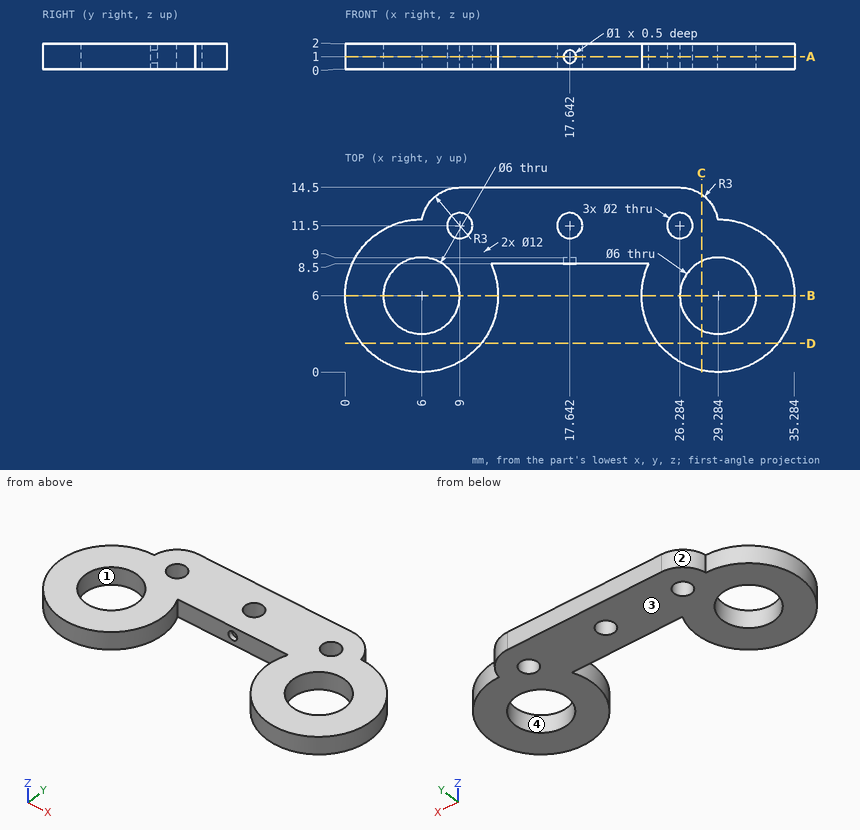
For this review, use the dimensioned drawing (mm, ordinates from the lowest corner) and the shaded views. Coordinates: 2 decimals unless noted, no trailing zeros. Loops run counter-clockwise (first coordinate to the right, second up) from the corner with the lowest first, then second, coordinate; pieces in that order, holes last.
1. Insertion check: P1, Ø5, axis at x = 29.28, y = 6, coming from the +Z side; P2, Ø0.6, axis at x = 20, z = 1.5, coming from the -Y side. Each pin has a flat end and moves straight along its axis. Give the tip position at first contact, or say it passes through.
2. For line 1 (Y direction, x = 29.5, z = 0.8); line 2 (X direction, y = 5, z = 1.6) (1 decimal); line 3 (Y direction, x = 31, z = 0.25), list the stretches that pass through material, from the lowest coordinate up.
3. Add section B-B, the plane y = 6. Give the boundary of the cut face in (x, z).
4. Add section D-D, the plane y = 2.25. Give the boundary of the cut face in (x, z).
5. Add section C-C, the plane x = 28. Give the boundary of the cut face in (y, z).
6. Add section A-A, the plane z = 1. Give the boundary of the cut face in (x, y).
7. Mouldability with a two-part tool opening along Y and no side actions: class the marked faces 1, 2, 3 and 4 as +Y half, -Y half, draft (parallel to the pull), parting line (faces both ways), or undercut.
Result:
1. P1: passes through
1. P2: stops at y = 8.5
2. line 1: y = 0 to 3.01, 8.99 to 12
2. line 2: x = 0.1 to 3.2, 8.8 to 11.9, 23.4 to 26.5, 32.1 to 35.2
2. line 3: y = 0.25 to 3.54, 8.46 to 11.75
3. outline: (0, 0) - (3, 0) - (3, 2) - (0, 2) - close; (9, 0) - (12, 0) - (12, 2) - (9, 2) - close; (23.28, 0) - (26.28, 0) - (26.28, 2) - (23.28, 2) - close; (32.28, 0) - (35.28, 0) - (35.28, 2) - (32.28, 2) - close
4. outline: (1.32, 0) - (10.68, 0) - (10.68, 2) - (1.32, 2) - close; (24.6, 0) - (33.97, 0) - (33.97, 2) - (24.6, 2) - close
5. outline: (0.14, 0) - (3.29, 0) - (3.29, 2) - (0.14, 2) - close; (8.71, 0) - (13.96, 0) - (13.96, 2) - (8.71, 2) - close
6. outline: (6.04, 12) arc R6 ccw (long way) to (11.45, 8.5) - (17.14, 8.5) - (17.14, 9) - (18.14, 9) - (18.14, 8.5) - (23.83, 8.5) arc R6 ccw (long way) to (29.24, 12) arc R3 ccw to (26.28, 14.5) - (9, 14.5) arc R3 ccw to start; hole circle Ø6 at (6, 6); hole circle Ø2 at (9, 11.5); hole circle Ø2 at (17.64, 11.5); hole circle Ø2 at (26.28, 11.5); hole circle Ø6 at (29.28, 6)
7. face 1: undercut
7. face 2: +Y half
7. face 3: draft
7. face 4: undercut
